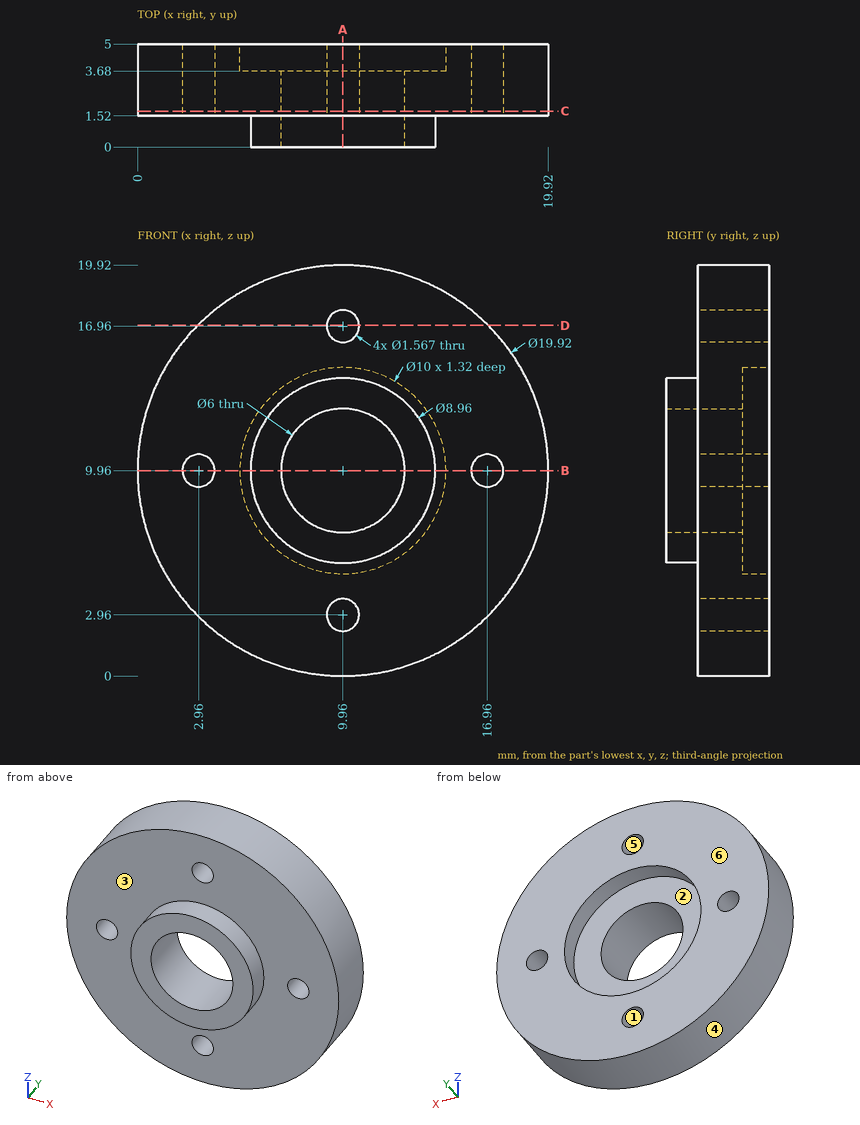
Print and shaded views of the part. All mm, measured from the part's lowest x, y and z. A direction names the side the tool comes from. Round coordinates to 2 decimals unless told otherwise and drop trailing zeros. Write each loop counter-clockwise with the first axis right and the second up, starting at its lowest first coordinate (ties: lowest second). Pieces come first, ordered by that corner, then holes. Notation, with made-up numbers: (9.25, -7.5) - (45.25, -7.5) arc R29 ccw to (45.25, 16.5) - close; hole circle Ø3 at (11, -37). An arc over 180 degrees is marked (long way). Write each question's results on one line, items separated by ' | '. Start each with the question number.
Item 1: Saw through at A-A (x = 9.96). Write the cut outline in (y, z), and give its area (3 significant figures).
Item 2: Drop flat-ended pins along their axis: P1, Ø2, axis at y = 4, z = 8, coming from the +X side; P2, Ø1, axis at y = 3, z = 14.5, coming from the +X side; P3, Ø2, axis at y = 3.5, z = 6.5, coming from the -X side. Give the stop position or say it passes through.
Item 3: Saw through at C-C (y = 1.75). Write the cut outline in (x, z), and give its area (3 significant figures).
Item 4: Saw through at D-D (z = 17). Write the cut outline in (x, y).
Item 5: Which spindle directions (+Z, -Z, +X, -X, +Y, -Y) get a long thin tool onto all of the face, cutting with end or side? Do the marked faces 1, 2 and 3. Say none if no direction does.
Item 6: Saw through at B-B (z = 9.96). Write the cut outline in (x, y), and give its area (3 significant figures).
Item 7: Mould opens along Z. For the marked faces 4, 5 and 6 say: pulls with the +Z half, pulls with the -Z half, needs draft (parallel to the pull), parting line crosses it, or undercut.
Item 8: Wall check: L1, parallel to Z at x = 9.96, y = 4.4; L2, parallel to Z at x = 9.96, y = 2.9; L3, parallel to Y at x = 6, z = 9.75. Give the ranges that are in metal, low to high. Write a range as [from, to].
Results are:
1) outline: (0, 5.48) - (1.52, 5.48) - (1.52, 3.74) - (5, 3.74) - (5, 4.96) - (3.68, 4.96) - (3.68, 6.96) - (0, 6.96) - close; (0, 12.96) - (3.68, 12.96) - (3.68, 14.96) - (5, 14.96) - (5, 16.18) - (1.52, 16.18) - (1.52, 14.44) - (0, 14.44) - close; (1.52, 0) - (5, 0) - (5, 2.18) - (1.52, 2.18) - close; (1.52, 17.74) - (5, 17.74) - (5, 19.92) - (1.52, 19.92) - close | area: 36.8 mm²
2) P1: stops at x = 19.87 | P2: stops at x = 19.06 | P3: stops at x = 0.31
3) outline: circle Ø19.92 at (9.96, 9.96); hole circle Ø1.57 at (2.96, 9.96); hole circle Ø6 at (9.96, 9.96); hole circle Ø1.57 at (9.96, 2.96); hole circle Ø1.57 at (9.96, 16.96); hole circle Ø1.57 at (16.96, 9.96) | area: 276 mm²
4) outline: (2.91, 1.52) - (9.18, 1.52) - (9.18, 5) - (2.91, 5) - close; (10.74, 1.52) - (17.01, 1.52) - (17.01, 5) - (10.74, 5) - close
5) face 1: +Y, -Y | face 2: +Y | face 3: -Y
6) outline: (0, 1.52) - (2.18, 1.52) - (2.18, 5) - (0, 5) - close; (3.74, 1.52) - (5.48, 1.52) - (5.48, 0) - (6.96, 0) - (6.96, 3.68) - (4.96, 3.68) - (4.96, 5) - (3.74, 5) - close; (12.96, 0) - (14.44, 0) - (14.44, 1.52) - (16.18, 1.52) - (16.18, 5) - (14.96, 5) - (14.96, 3.68) - (12.96, 3.68) - close; (17.74, 1.52) - (19.92, 1.52) - (19.92, 5) - (17.74, 5) - close | area: 36.8 mm²
7) face 4: parting line crosses it | face 5: undercut | face 6: needs draft
8) L1: z = [0, 2.18], [3.74, 4.96], [14.96, 16.18], [17.74, 19.92] | L2: z = [0, 2.18], [3.74, 6.96], [12.96, 16.18], [17.74, 19.92] | L3: y = [0, 3.68]
